from build123d import *

# Parameters (mm, degrees)
BOSS_EXTRUDE1_DEPTH = 6
SKETCH3_R           = 1.55
CUT_EXTRUDE1_DEPTH  = 17.911534525
SKETCH5_R           = 1.55
CUT_EXTRUDE2_DEPTH  = 21.05617112


with BuildPart() as part:
    # Sketch1 → Boss-Extrude1 (new body)
    with BuildSketch(Plane.XY):
        Polygon((3.5, -6), (0.5, -6), (-6.5, -6), (-6.5, -9), (6.5, -9), (6.5, 9), (3.5, 9), (3.5, -4.7), align=None)
    extrude(amount=BOSS_EXTRUDE1_DEPTH)

    # Sketch3 → Cut-Extrude1 (cut, through all)
    with BuildSketch(Plane(origin=(6.5, 0, 0), x_dir=(0, 0, -1), z_dir=(1, 0, 0))):
        with Locations(Location((-3, 6, 0), (0, 0, 90))):
            Circle(SKETCH3_R)
        with Locations(Location((-3, -2, 0), (0, 0, 90))):
            Circle(SKETCH3_R)
    extrude(amount=-CUT_EXTRUDE1_DEPTH, mode=Mode.SUBTRACT)

    # Sketch5 → Cut-Extrude2 (cut, through all)
    with BuildSketch(Plane.XZ.offset(9)):
        with Locations(Location((-3.5, 3, 0), (0, 0, 270))):
            Circle(SKETCH5_R)
    extrude(amount=-CUT_EXTRUDE2_DEPTH, mode=Mode.SUBTRACT)


solid = part.part
Design review of the part built by this model. Coordinates are the model's own, in mm. A direction names the side the tool comes from. Coordinates: 2 decimals unless noted, no trailing zeros. Order: outer loops, then holes, each group sorted by start corner. A loop starts at its lowest first (then second) coordinate and runs counter-clockwise, first axis right, second up.
Item 1: For faces 1 (the flat face through (3.5, 2, 3)), 2 (the flat face through (4, -3, 0)), list the 3-axis set-ups (+Z, -Z, +X, -X, +Y, -Y) from which the entire face can be reached by the end or side of a thin tool; tool diameter is ignored.
Item 2: For pin 1 Ø1.8 at (y, z) = (3, 2) entering from -X; pin 2 Ø3 at (x, z) = (-3.5, 3) entering from -Y; pin 3 Ø3 at (x, z) = (-2.5, 2.5) entering from +Y, all flat-tipped, find the tip position at first contact; note any pin that passes through.
Item 3: For line 1 (Z direction, x = 4.5, y = -2); line 2 (X direction, y = -8.3, z = 3); line 3 (Y direction, x = 4.25, z = 1.95), list the stretches that pass through material, from the lowest coordinate up.
Item 4: Take a section at B-B, the plane y = 6. Write out the cut boundary in (x, z), then the cut area to 3 significant figures.
Item 5: Take a section at C-C, the plane z = 3. Write out the cut boundary in (x, y).
Item 6: The part is to be moulded in two halves that separate along X. For faces 3 (the flat face through (0, -9, 3)), 4 (the cylindrical face through (-2.45, -7.52, 4.14)), 5 (the flat face through (6.5, 0, 3)), say which applies: pulls with the +X half, pulls with the -X half, needs draft (parallel to the pull), parting line crosses it, or undercut.
Item 7: Take a section at D-D, the plane x = 3.75. Write out the cut boundary in (y, z), then the cut area to 3 significant figures.
Item 8: Take a section at A-A, the plane x = -3.5. Write out the cut boundary in (y, z), then the cut area to 3 significant figures.
The answers:
1. face 1: +Z, -Z, -X, +Y
1. face 2: -Z, +X, -X, +Y, -Y
2. pin 1: stops at x = 3.5
2. pin 2: passes through
2. pin 3: stops at y = -6
3. line 1: z = 0 to 1.45, 4.55 to 6
3. line 2: x = -6.5 to -5.05, -1.95 to 6.5
3. line 3: y = -9 to -3.14, -0.86 to 4.86, 7.14 to 9
4. outline: (3.5, 0) - (6.5, 0) - (6.5, 1.45) - (3.5, 1.45) - close; (3.5, 4.55) - (6.5, 4.55) - (6.5, 6) - (3.5, 6) - close
4. area: 8.70 mm2
5. outline: (-6.5, -9) - (-5.05, -9) - (-5.05, -6) - (-6.5, -6) - close; (-1.95, -9) - (6.5, -9) - (6.5, -3.55) - (3.5, -3.55) - (3.5, -6) - (-1.95, -6) - close; (3.5, -0.45) - (6.5, -0.45) - (6.5, 4.45) - (3.5, 4.45) - close; (3.5, 7.55) - (6.5, 7.55) - (6.5, 9) - (3.5, 9) - close
6. face 3: needs draft
6. face 4: undercut
6. face 5: pulls with the +X half
7. outline: (-9, 0) - (9, 0) - (9, 6) - (-9, 6) - close; hole circle Ø3.1 at (-2, 3); hole circle Ø3.1 at (6, 3)
7. area: 92.9 mm2
8. outline: (-9, 0) - (-6, 0) - (-6, 1.45) - (-9, 1.45) - close; (-9, 4.55) - (-6, 4.55) - (-6, 6) - (-9, 6) - close
8. area: 8.70 mm2
